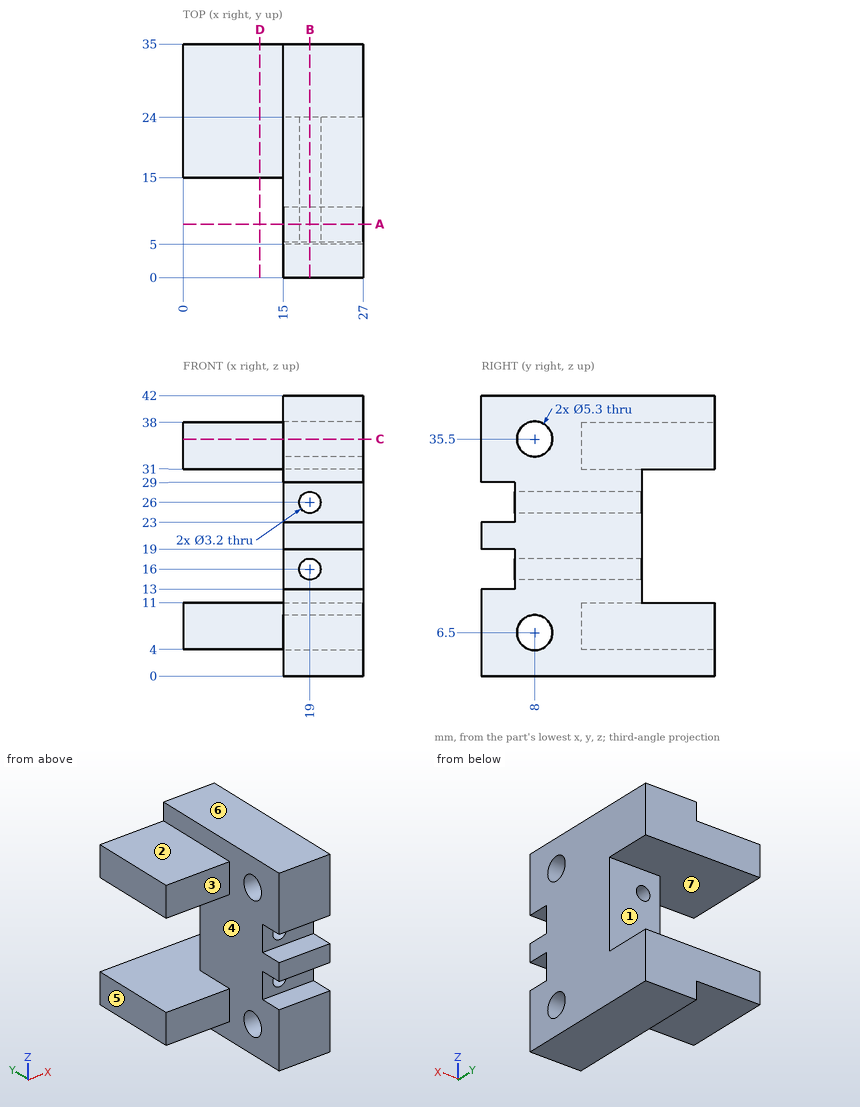
Geometry: see drawing. Coordinates: mm, zero at the bounding-box minimum. A direction names the side the tool comes from. Round coordinates to 2 decimals unless told otherwise and drop trailing zeros. Write each loop counter-clockwise with the first axis right and the second up, starting at its lowest first coordinate (ties: lowest second). Pieces come first, ordered by that corner, then holes. Notation, with made-up numbers: (36.25, 22) - (57.25, 22) arc R24 cw to (57.25, 50) - close; hole circle Ø4 at (-25, -31.75). An arc over 180 degrees is marked (long way). Use CSV: the item, a comma, the result in double quotes. Start each with the question number.
(1) Cut plane D-D, the plane x = 11.5. Return loops of the section in (y, z).
(2) Cut plane B-B, the plane x = 19. Return loops of the section in (y, z).
(3) Cut plane A-A, the plane y = 8. Return loops of the section in (x, z).
(4) Set-up query: the marked faces 1, 2 and 3. Return all of +Z, -Z, +X, -X, +Y, -Y with unobstructed straight access to the full face (end or side cutting, diameter ignored); none if empty.
(5) Cut plane C-C, the plane z = 35.5. Return loops of the section in (x, y).
(6) Material intervals for probe 1 along Z at (x, y) = (24, 8); probe 2 along Z at (x, y) = (19, 13); probe 3 along Y at (x, z) = (22, 35.5), sorted ascending. Write a range as [from, to].
(7) Mould query, pull axis Z, two halves, no side actions, for the marked faces 4, 5, 6 and 7. Classes: pulls with the +Z half, pulls with the -Z half, needs draft (parallel to the pull), parting line crosses it, or undercut.
(8) First-contact query: pin 1 Ø4 at (y, z) = (12.5, 25.5) entering from -X; pin 2 Ø10 at (x, y) = (9, 25) entering from -Z; pin 3 Ø7.5 at (x, z) = (6, 36) entering from -Y; pin 4 Ø1.9 at (x, z) = (19, 26) entering from -Y. Flat tips, straight axial feed; report the tip coordinate or a pass-through.
Geometry says:
1,outline,"(15, 4) - (35, 4) - (35, 11) - (15, 11) - close; (15, 31) - (35, 31) - (35, 38) - (15, 38) - close"
2,outline,"(0, 0) - (35, 0) - (35, 11) - (24, 11) - (24, 14.4) - (5, 14.4) - (5, 13) - (0, 13) - close; (0, 19) - (5, 19) - (5, 17.6) - (24, 17.6) - (24, 24.4) - (5, 24.4) - (5, 23) - (0, 23) - close; (0, 29) - (5, 29) - (5, 27.6) - (24, 27.6) - (24, 31) - (35, 31) - (35, 42) - (0, 42) - close; hole circle Ø5.3 at (8, 6.5); hole circle Ø5.3 at (8, 35.5)"
3,outline,"(15, 0) - (27, 0) - (27, 3.85) - (15, 3.85) - close; (15, 9.15) - (27, 9.15) - (27, 32.85) - (15, 32.85) - close; (15, 38.15) - (27, 38.15) - (27, 42) - (15, 42) - close; hole circle Ø3.2 at (19, 16); hole circle Ø3.2 at (19, 26)"
4,face 1,"+X, -X, +Y"
4,face 2,"+Z, -X, +Y, -Y"
4,face 3,"+Z, -Z, -X, -Y"
5,outline,"(0, 15) - (15, 15) - (15, 10.65) - (27, 10.65) - (27, 35) - (0, 35) - close; (15, 0) - (27, 0) - (27, 5.35) - (15, 5.35) - close"
6,probe 1,"[0, 3.85], [9.15, 32.85], [38.15, 42]"
6,probe 2,"[0, 14.4], [17.6, 24.4], [27.6, 42]"
6,probe 3,"[0, 5.35], [10.65, 35]"
7,face 4,"undercut"
7,face 5,"needs draft"
7,face 6,"pulls with the +Z half"
7,face 7,"undercut"
8,pin 1,"x = 15"
8,pin 2,"z = 4"
8,pin 3,"y = 15"
8,pin 4,"through"
